```python
from build123d import *

# Parameters (mm, degrees)
CROQUIS1_R              = 8.6
SALIENTE_EXTRUIR1_DEPTH = 12.5
CROQUIS3_W              = 23.2
CROQUIS3_H              = 25
CROQUIS3_R              = 8.6
SALIENTE_EXTRUIR2_DEPTH = 25


with BuildPart() as part:
    # Croquis1 → Saliente-Extruir1 (new, symmetric)
    with BuildSketch(Plane.XY):
        with BuildLine():
            Line((-11.6, -10), (11.6, -10))
            Line((11.6, -10), (11.6, 0))
            ThreePointArc((11.6, 0), (0, 11.6), (-11.6, 0))
            Line((-11.6, 0), (-11.6, -10))
        make_face()
        Circle(CROQUIS1_R, mode=Mode.SUBTRACT)
    extrude(amount=SALIENTE_EXTRUIR1_DEPTH, both=True)

    # Croquis3 → Saliente-Extruir2 (add)
    with BuildSketch(Plane(origin=(0, -10, 0), x_dir=(-1, 0, 0), z_dir=(0, -1, 0))):
        Rectangle(CROQUIS3_W, CROQUIS3_H)
        with Locations(Location((0, 0, 0), (0, 0, 90))):
            Circle(CROQUIS3_R, mode=Mode.SUBTRACT)
    extrude(amount=SALIENTE_EXTRUIR2_DEPTH)


solid = part.part
```
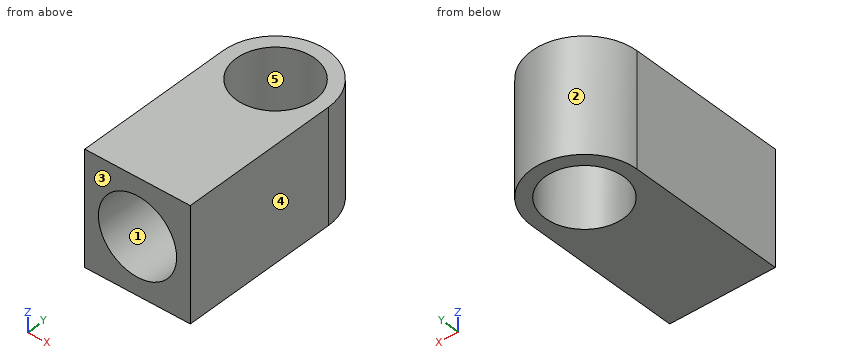
Here's how the part is built. I have some questions about the finished solid (model axes, mm). Face numbers are marked on the shaded views. A direction names the side the tool comes from. Round coordinates to 2 decimals unless told otherwise and drop trailing zeros. Loops run counter-clockwise (first coordinate to the right, second up) from the corner with the lowest first, then second, coordinate; pieces in that order, holes last.
1. Suppose I cut it at A-A, the plane x = 0. Please give me the cut outline in (y, z), and give its area (3 significant figures).
Answers:
outline: (-35, -12.5) - (-8.6, -12.5) - (-8.6, 12.5) - (-35, 12.5) - (-35, 8.6) - (-10, 8.6) - (-10, -8.6) - (-35, -8.6) - close; (8.6, -12.5) - (11.6, -12.5) - (11.6, 12.5) - (8.6, 12.5) - close
area: 305 mm2
2. Suppose I cut it at D-D, the plane y = -20. Please give me the cut outline in (x, z).
Answers:
outline: (-11.6, -12.5) - (11.6, -12.5) - (11.6, 12.5) - (-11.6, 12.5) - close; hole circle Ø17.2 at (0, 0)
3. Will this pin go through, and if not, where does the flat tip stop? pin 1 (2 mm diameter, centred on x = -2.5, z = 0, fed in from -Y).
Answers:
pin 1: stops at y = -10
4. Suppose I cut it at B-B, the plane z = 0. Please give me the cut outline in (x, y).
Answers:
outline: (-11.6, -35) - (-8.6, -35) - (-8.6, -10) - (8.6, -10) - (8.6, -35) - (11.6, -35) - (11.6, 0) arc R11.6 ccw to (-11.6, 0) - close; hole circle Ø17.2 at (0, 0)
5. Suppose I cut it at C-C, the plane y = 5.5. Please give me the cut outline in (x, z), and give its area (3 significant figures).
Answers:
outline: (-10.21, -12.5) - (-6.61, -12.5) - (-6.61, 12.5) - (-10.21, 12.5) - close; (6.61, -12.5) - (10.21, -12.5) - (10.21, 12.5) - (6.61, 12.5) - close
area: 180 mm2
6. Thinking about a two-plate mould opening in X: for the marked faces 3, 4 and 5, which applies, released by +X, released by -X, zero draft, split by the parting line, or undercut?
Answers:
face 3: zero draft
face 4: released by +X
face 5: undercut
7. If I drill on probe 1 along Y at (x, z) = (0, -5); probe 2 along X at (y, z) = (-25, -0.25); probe 3 along X at (y, z) = (-18, 3.5), over which ranges is the centre line in solid material (lowest first)?
Answers:
probe 1: y = -10 to -8.6, 8.6 to 11.6
probe 2: x = -11.6 to -8.6, 8.6 to 11.6
probe 3: x = -11.6 to -7.86, 7.86 to 11.6
8. For the marked faces 1 and 2, which set-ups out of +Z, -Z, +X, -X, +Y, -Y let a thin tool reach every point of the face, with its end or its side?
Answers:
face 1: -Y
face 2: +Z, -Z, +Y
